Geometry check sheet. Reference: the model listing, model coordinates, mm. A direction names the side the tool comes from. Coordinates: 2 decimals unless noted, no trailing zeros. Write each loop counter-clockwise with the first axis right and the second up, starting at its lowest first coordinate (ties: lowest second). Pieces come first, ordered by that corner, then holes. Notation, with made-up numbers: (46.5, 68.5) -> (85.5, 68.5) arc R15 ccw to (85.5, 85.5) -> close; hole circle Ø8 at (-12, 77.5). An arc over 180 degrees is marked (long way). Answer in a Markdown table with one row per item. Add a question column.
Q1. Gauge pin test, flat ends, axial feed: P1, Ø8.5, axis at x = 4, z = -66, coming from the +Y side; P2, Ø2, axis at y = 5, z = -59, coming from the +X side; P3, Ø8, axis at y = 9.5, z = 10.5, coming from the +X side. Record the tip position at first contact, or that the pin passes through.
Q2. Thickness scan on line 1 (Y direction, x = -2.75, z = -43); line 2 (X direction, y = -7.75, z = 7.5). Record the ranges inside material, lowest first.
Q3. Tool access check on faces 1 (the face through (-1.396, -4, -36)), 2 (the face through (1.396, -4, -36)), 3 (the face through (9.05, 0.02, -10.64)). Record the directions out of +Z, -Z, +X, -X, +Y, -Y that give a thin tool (end or side, any length) a straight path to the whole face; none if there is none.
Q4. Section check A-A, the plane z = -16. Record the boundary of the cut face in (x, y), and give its area (3 significant figures).
```python
from build123d import *

# Parameters (mm, degrees)
F0_R      = 12.5
F1_DEPTH  = 17.5
F2_R      = 2
F3_R      = 12.5
F4_DEPTH  = 2
F5_R      = 9.05
F6_DEPTH  = 100
F8_ANGLE  = 180
F10_DEPTH = 100.001
F12_DEPTH = 15


with BuildPart() as f1:
    # F0 (on Top) → F1 (new body)
    with BuildSketch(Plane.XY):
        Circle(F0_R)
    extrude(amount=F1_DEPTH)

    # F2
    f2_edges = [f1.edges().sort_by_distance(p)[0] for p in [
        (-12.5, 0, 17.5),
    ]]
    fillet(f2_edges, radius=F2_R)

    # F3 (on face) → F4 (join)
    with BuildSketch(Plane(origin=(0, 0, 0), x_dir=(1, 0, 0), z_dir=(0, 0, -1))):
        Circle(F3_R)
    extrude(amount=F4_DEPTH)

    # F5 (on face) → F6 (join)
    with BuildSketch(Plane(origin=(0, 0, -2), x_dir=(1, 0, 0), z_dir=(0, 0, -1))):
        Circle(F5_R)
    extrude(amount=F6_DEPTH)

    # F7 (on Front) → F8 (revolve, cut)
    with BuildSketch(Plane.XZ):
        with BuildLine():
            Line((-9.05, -19.527881), (-9.05, -2))
            ThreePointArc((-9.05, -2), (-9.133447, -10.763941), (-9.05, -19.527881))
        make_face()
        with BuildLine():
            Line((9.05, -2), (9.05, -19.527881))
            ThreePointArc((9.05, -19.527881), (9.133447, -10.763941), (9.05, -2))
        make_face()
        with BuildLine():
            ThreePointArc((9.05, -19.527881), (6.387127, -60.968279), (0, -102))
            Line((0, -102), (9.05, -102))
            Line((9.05, -102), (9.05, -19.527881))
        make_face()
        with BuildLine():
            ThreePointArc((0, -102), (-6.387127, -60.968279), (-9.05, -19.527881))
            Line((-9.05, -19.527881), (-9.05, -102))
            Line((-9.05, -102), (0, -102))
        make_face()
    revolve(axis=Axis((0, 0, -52), (0, 0, -1)), revolution_arc=F8_ANGLE, mode=Mode.SUBTRACT)

    # F9 (on face) → F10 (cut, through all)
    with BuildSketch(Plane(origin=(0, 0, -2), x_dir=(1, 0, 0), z_dir=(0, 0, -1))):
        Polygon((-1.395766, -12.419861), (-1.395766, -7.419861), (-1.395766, -1.395766), (-7.419861, -1.395766), (-12.419861, -1.395766), align=None)
        Polygon((-12.419861, 1.395766), (-7.419861, 1.395766), (-1.395766, 1.395766), (-1.395766, 7.419861), (-1.395766, 12.419861), align=None)
        Polygon((1.395766, 12.419861), (1.395766, 7.419861), (1.395766, 1.395766), (7.419861, 1.395766), (12.419861, 1.395766), align=None)
        Polygon((12.419861, -1.395766), (7.419861, -1.395766), (1.395766, -1.395766), (1.395766, -7.419861), (1.395766, -12.419861), align=None)
    extrude(amount=F10_DEPTH, mode=Mode.SUBTRACT)

    # F11 (on face) → F12 (cut)
    with BuildSketch(Plane.XY.offset(17.5)):
        with BuildLine():
            Line((-2.5, -2.5), (-10.198039, -2.5))
            ThreePointArc((-10.198039, -2.5), (-7.424621, -7.424621), (-2.5, -10.198039))
            Line((-2.5, -10.198039), (-2.5, -2.5))
        make_face()
        with BuildLine():
            ThreePointArc((-2.5, -10.198039), (-7.424621, -7.424621), (-10.198039, -2.5))
            Line((-10.198039, -2.5), (-12.067753, -2.5))
            Line((-12.067753, -2.5), (-13.370921, -2.5))
            ThreePointArc((-13.370921, -2.5), (-9.618512, -9.618512), (-2.5, -13.370921))
            Line((-2.5, -13.370921), (-2.5, -10.63198))
            Line((-2.5, -10.63198), (-2.5, -10.198039))
        make_face()
        with BuildLine():
            ThreePointArc((10.198039, 2.5), (7.424621, 7.424621), (2.5, 10.198039))
            Line((2.5, 10.198039), (2.5, 2.5))
            Line((2.5, 2.5), (10.198039, 2.5))
        make_face()
        with BuildLine():
            Line((2.5, 10.63198), (2.5, 10.198039))
            ThreePointArc((2.5, 10.198039), (7.424621, 7.424621), (10.198039, 2.5))
            Line((10.198039, 2.5), (10.63198, 2.5))
            Line((10.63198, 2.5), (13.370921, 2.5))
            ThreePointArc((13.370921, 2.5), (9.618512, 9.618512), (2.5, 13.370921))
            Line((2.5, 13.370921), (2.5, 10.63198))
        make_face()
        with BuildLine():
            ThreePointArc((2.5, -10.198039), (7.424621, -7.424621), (10.198039, -2.5))
            Line((10.198039, -2.5), (2.5, -2.5))
            Line((2.5, -2.5), (2.5, -10.198039))
        make_face()
        with BuildLine():
            Line((10.63198, -2.5), (10.198039, -2.5))
            ThreePointArc((10.198039, -2.5), (7.424621, -7.424621), (2.5, -10.198039))
            Line((2.5, -10.198039), (2.5, -10.63198))
            Line((2.5, -10.63198), (2.5, -13.370921))
            ThreePointArc((2.5, -13.370921), (9.618512, -9.618512), (13.370921, -2.5))
            Line((13.370921, -2.5), (10.63198, -2.5))
        make_face()
        with BuildLine():
            Line((-2.5, 10.198039), (-2.5, 10.63198))
            Line((-2.5, 10.63198), (-2.5, 13.370921))
            ThreePointArc((-2.5, 13.370921), (-9.618512, 9.618512), (-13.370921, 2.5))
            Line((-13.370921, 2.5), (-10.63198, 2.5))
            Line((-10.63198, 2.5), (-10.198039, 2.5))
            ThreePointArc((-10.198039, 2.5), (-7.424621, 7.424621), (-2.5, 10.198039))
        make_face()
        with BuildLine():
            Line((-2.5, 2.5), (-2.5, 10.198039))
            ThreePointArc((-2.5, 10.198039), (-7.424621, 7.424621), (-10.198039, 2.5))
            Line((-10.198039, 2.5), (-2.5, 2.5))
        make_face()
    extrude(amount=-F12_DEPTH, mode=Mode.SUBTRACT)


solid = f1.part
```
Calculated:
| question | item | result |
|---|---|---|
| 1 | P1 | stops at y = 6.08 |
| 1 | P2 | stops at x = 1.4 |
| 1 | P3 | stops at x = 2.5 |
| 2 | line 1 | y = -1.4 to 1.4 |
| 2 | line 2 | x = -2.5 to 2.5 |
| 3 | face 1 | -Z, -X, -Y |
| 3 | face 2 | -Z, +X, -Y |
| 3 | face 3 | -Z, +X |
| 4 | outline | (-8.94, -1.4) -> (-1.4, -1.4) -> (-1.4, -8.94) arc R9.05 ccw to (1.4, -8.94) -> (1.4, -1.4) -> (8.94, -1.4) arc R9.05 ccw to (8.94, 1.4) -> (1.4, 1.4) -> (1.4, 8.94) arc R9.05 ccw to (-1.4, 8.94) -> (-1.4, 1.4) -> (-8.94, 1.4) arc R9.05 ccw to start |
| 4 | area | 92.9 mm² |
